Part print with two shaded views. Sizes in mm from the minimum x, y, z corner. Round coordinates to 2 decimals unless told otherwise and drop trailing zeros. Write each loop counter-clockwise with the first axis right and the second up, starting at its lowest first coordinate (ties: lowest second). Pieces come first, ordered by that corner, then holes.
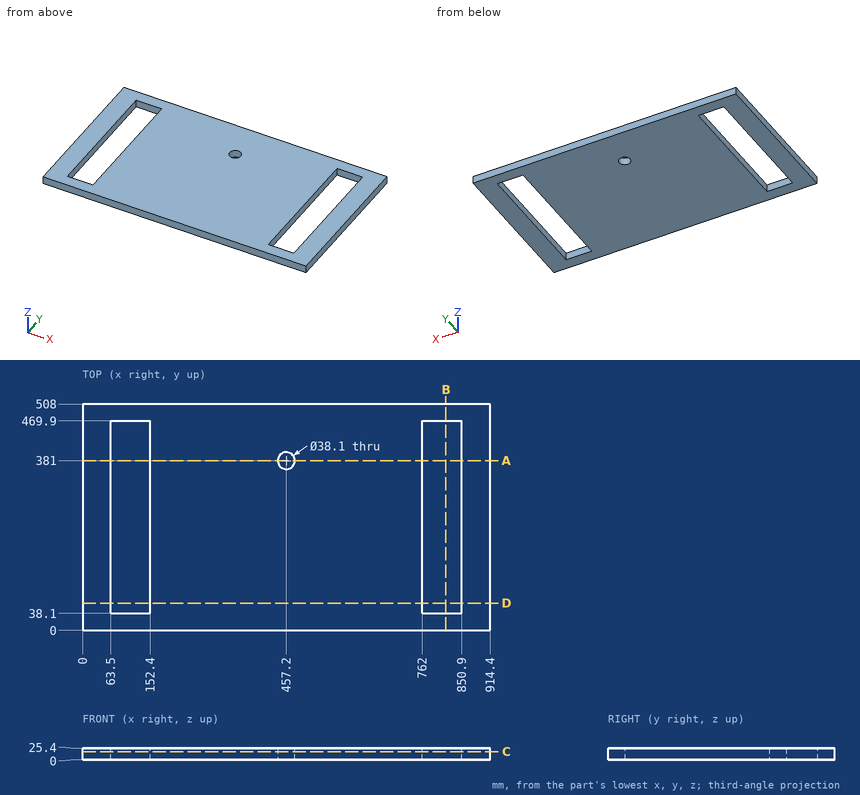
Q1. Cut at C-C on z = 18. Write the cut outline in (x, y).
Values follow:
outline: (0, 0) - (914.4, 0) - (914.4, 508) - (0, 508) - close; hole (63.5, 38.1) - (152.4, 38.1) - (152.4, 469.9) - (63.5, 469.9) - close; hole circle Ø38.1 at (457.2, 381); hole (762, 38.1) - (850.9, 38.1) - (850.9, 469.9) - (762, 469.9) - close
Q2. Cut at B-B on x = 815.5. Write the cut outline in (y, z), plus the area to 3 significant figures.
Values follow:
outline: (0, 0) - (38.1, 0) - (38.1, 25.4) - (0, 25.4) - close; (469.9, 0) - (508, 0) - (508, 25.4) - (469.9, 25.4) - close
area: 1,940 mm2
Q3. Wall check: L1, parallel to X at y = 207.5, z = 15.75; L2, parallel to Y at x = 812, z = 14; L3, parallel to Y at x = 457.2, z = 11. Give the ranges that are in metal, low to high.
Values follow:
L1: x = 0 to 63.5, 152.4 to 762, 850.9 to 914.4
L2: y = 0 to 38.1, 469.9 to 508
L3: y = 0 to 361.95, 400.05 to 508
Q4. Cut at A-A on y = 381. Write the cut outline in (x, z), plus the area to 3 significant figures.
Values follow:
outline: (0, 0) - (63.5, 0) - (63.5, 25.4) - (0, 25.4) - close; (152.4, 0) - (438.15, 0) - (438.15, 25.4) - (152.4, 25.4) - close; (476.25, 0) - (762, 0) - (762, 25.4) - (476.25, 25.4) - close; (850.9, 0) - (914.4, 0) - (914.4, 25.4) - (850.9, 25.4) - close
area: 17,700 mm2
Q5. Cut at D-D on y = 61. Write the cut outline in (x, z).
Values follow:
outline: (0, 0) - (63.5, 0) - (63.5, 25.4) - (0, 25.4) - close; (152.4, 0) - (762, 0) - (762, 25.4) - (152.4, 25.4) - close; (850.9, 0) - (914.4, 0) - (914.4, 25.4) - (850.9, 25.4) - close
